Autodesk Inventor part; units mm, degrees
ref_plane "YZ Plane" through (0, 0, 0) normal (1, 0, 0) x (0, 1, 0)
ref_plane "XZ Plane" through (0, 0, 0) normal (0, 1, 0) x (-1, 0, 0)
ref_plane "XY Plane" through (0, 0, 0) normal (0, 0, 1) x (1, 0, 0)
sketch "Sketch1" plane through (0, 0, 0) normal (0, 0, 1) x (1, 0, 0)
  line L0 (-21, 0) -> (21, 0) construction
  line L1 (0, -140) -> (0, 140) construction
  line L2 (-15, 100) -> (15, 100)
  line L3 (15, 100) -> (15, -100)
  line L4 (15, -100) -> (-15, -100)
  line L5 (-15, -100) -> (-15, 100)
  line L6 (-0.1, 90.05) -> (15, 90.05)
  line L7 (15, 90.05) -> (15, -100)
  line L8 (15, -100) -> (-0.1, -100)
  line L9 (-0.1, -100) -> (-0.1, 90.05)
  circle A0 centre (1.9, 88.05) radius 3
  line L10 (9.9, 100) -> (15, 100)
  line L11 (15, 100) -> (15, 90.05)
  line L12 (15, 90.05) -> (9.9, 90.05)
  line L13 (9.9, 90.05) -> (9.9, 100)
  point P0 (0, 0)
  point P1 (15, 90.05)
  point P2 (4.1361, 90.05)
  point P3 (-0.1, 85.8139)
  dimension "d0" = 30
  dimension "d1" = 200
  dimension "d2" = 9.95
  dimension "d3" = 15.1
  dimension "d16" = 2
  dimension "d17" = 6
  dimension "d18" = 2
  dimension "d23" = 14.9
  dimension "d27" = 10
extrude "Extrusion1" add sketch "Sketch1" against normal blind 10
extrude "Extrusion2" cut sketch "Sketch1" against normal blind 6.1 contours L2 L3 L6 L13 | L6 L3 L4 L9 A0 | A0 L9 L6 | L6 L9 A0
sketch "Sketch2" plane through (0, 0, -10) normal (0, 0, -1) x (-1, 0, 0)
  line L0 (-4.1361, 90.05) -> (-9.9, 90.05) construction
  line L1 (-9.9, 100) -> (15, 100) construction
  line L2 (15, 100) -> (15, -100) construction
  line L3 (15, -100) -> (0.1, -100) construction
  line L4 (0.1, -100) -> (0.1, 85.8139) construction
  line L5 (7.5, -100) -> (7.5, 100) construction
  line L6 (21, 0) -> (-21, 0) construction
  arc A0 (0.1, 85.8139) -> (-4.1361, 90.05) centre (-1.9, 88.05) ccw
  line L7 (-9.9, 90.05) -> (-9.9, 100)
  point P0 (0, 0)
  point P1 (7.5, -90)
  point P2 (7.5, 90)
  point P3 (7.5, 0)
  dimension "d8" = 180
  dimension "d25" = 7.5
hole "Hole1" at (-7.5, -90, -10) at (-7.5, 0, -10) at (-7.5, 90, -10) direction (0, 0, 1) diameter 4.5 end through all counterbore diameter 8 counterbore depth 4.6
fillet "Fillet1" radius 2 6 edges at (-15, -100, -5) (-15, 100, -5) (-0.1, -100, -3.05) (-0.1, 85.8139, -3.05) (4.1361, 90.05, -3.05) (9.9, 90.05, -3.05)
fillet "Fillet1" radius 1 3 edges at (15, -100, -8.05) (15, 100, -8.05) (9.9, 100, -3.05)
equation "\"d16\" = 0.333333 * d17"
equation "\"d18\" = d16"
properties part number "DLT-01-233" material "Acrílico TP"
Check sheet for the modelled part. Datum: model origin and axes. Units: mm. A direction names the side the tool comes from. Coordinates: 2 decimals unless noted, no trailing zeros. Write each loop counter-clockwise with the first axis right and the second up, starting at its lowest first coordinate (ties: lowest second). Pieces come first, ordered by that corner, then holes. Notation, with made-up numbers: M -38,81.5 L 9,81.5 A27 ccw 9,114.5 Z; hole C 88.25,61 d8. An arc over 180 degrees is marked long. Write item = value, one per line. Start each with the question number.
1. Sectioned sample at A-A (y = 0). Record the cut outline in (x, z), then the cut area to 3 significant figures.
2. Mould release check, pull along X, two halves, no side actions. Record for faces 1 (the flat face through (15, 1, -8)), 2 (the cylindrical face through (-8.176, -87.854, -2.662)), 3 (the flat face through (-5, 1, 0)), 4 (the cylindrical face through (-9.397, 1.21, -2.662)): pulls with the +X half, pulls with the -X half, needs draft (parallel to the pull), parting line crosses it, or undercut.
3. Sectioned sample at C-C (x = 2). Record the cut outline in (y, z).
4. Sectioned sample at B-B (x = -7.5). Record the cut outline in (y, z).
5. Thickness scan on probe 1 along Y at (x, z) = (-7.5, -2.25); probe 2 along Y at (x, z) = (-7.5, -6.55); probe 3 along X at (y, z) = (-90, -7.35). Record the ranges inside material, lowest first.
6. Go/stop test with flat-tipped pins: pin 1 (9 mm diameter, centred on x = -8.5, y = 88.5, fed in from -Z); pin 2 (1.5 mm diameter, centred on x = 6, z = -1.5, fed in from -Y); pin 3 (6.5 mm diameter, centred on x = -7.5, y = 90, fed in from -Z); pin 4 (1 mm diameter, centred on x = 8, y = 30.5, fed in from +Z). Record where each tip stops, or that it passes through.
7. Tool access check on faces 5 (the cylindrical face through (-0.18, 90.21, -3.01)), 6 (the flat face through (-6, 2, -5.4)), 7 (the flat face through (9.9, 95, -3)), 8 (the flat face through (-0.1, -8, -3)). Record the directions out of +Z, -Z, +X, -X, +Y, -Y that give a thin tool (end or side, any length) a straight path to the whole face; none if there is none.
The answers:
q1.outline = M -15,-10 L -11.5,-10 L -11.5,-5.4 L -9.75,-5.4 L -9.75,0 L -15,0 Z; M -5.25,-5.4 L -3.5,-5.4 L -3.5,-10 L 15,-10 L 15,-6.1 L -0.1,-6.1 L -0.1,0 L -5.25,0 Z
q1.area = 147 mm²
q2.face_1 = pulls with the +X half
q2.face_2 = undercut
q2.face_3 = needs draft
q2.face_4 = undercut
q3.outline = M -100,-10 L 100,-10 L 100,0 L 91.05,0 L 91.05,-6.1 L -100,-6.1 Z
q4.outline = M -100,-10 L -94,-10 L -94,-5.4 L -92.25,-5.4 L -92.25,0 L -100,0 Z; M -87.75,-5.4 L -86,-5.4 L -86,-10 L -4,-10 L -4,-5.4 L -2.25,-5.4 L -2.25,0 L -87.75,0 Z; M 2.25,-5.4 L 4,-5.4 L 4,-10 L 86,-10 L 86,-5.4 L 87.75,-5.4 L 87.75,0 L 2.25,0 Z; M 92.25,-5.4 L 94,-5.4 L 94,-10 L 100,-10 L 100,0 L 92.25,0 Z
q5.probe_1 = -100 to -92.25, -87.75 to -2.25, 2.25 to 87.75, 92.25 to 100
q5.probe_2 = -100 to -94, -86 to -4, 4 to 86, 94 to 100
q5.probe_3 = -15 to -11.5, -3.5 to 15
q6.pin_1 = -10
q6.pin_2 = 90.05
q6.pin_3 = -5.4
q6.pin_4 = -6.1
q7.face_5 = +Z
q7.face_6 = -Z
q7.face_7 = +Z, +X, +Y, -Y
q7.face_8 = +Z, +X, -Y
